Could you check a few things on this drawing? It's one solid part, dimensions in mm from its lowest x, y, z. Round coordinates to 2 decimals unless told otherwise and drop trailing zeros. Write each loop counter-clockwise with the first axis right and the second up, starting at its lowest first coordinate (ties: lowest second). Pieces come first, ordered by that corner, then holes. Notation, with made-up numbers: (26, 24.25) -> (43, 24.25) arc R25 ccw to (43, 44.25) -> close; hole circle Ø3 at (-37.5, -1). An arc over 180 degrees is marked (long way). Answer in a Markdown table with one row per item.
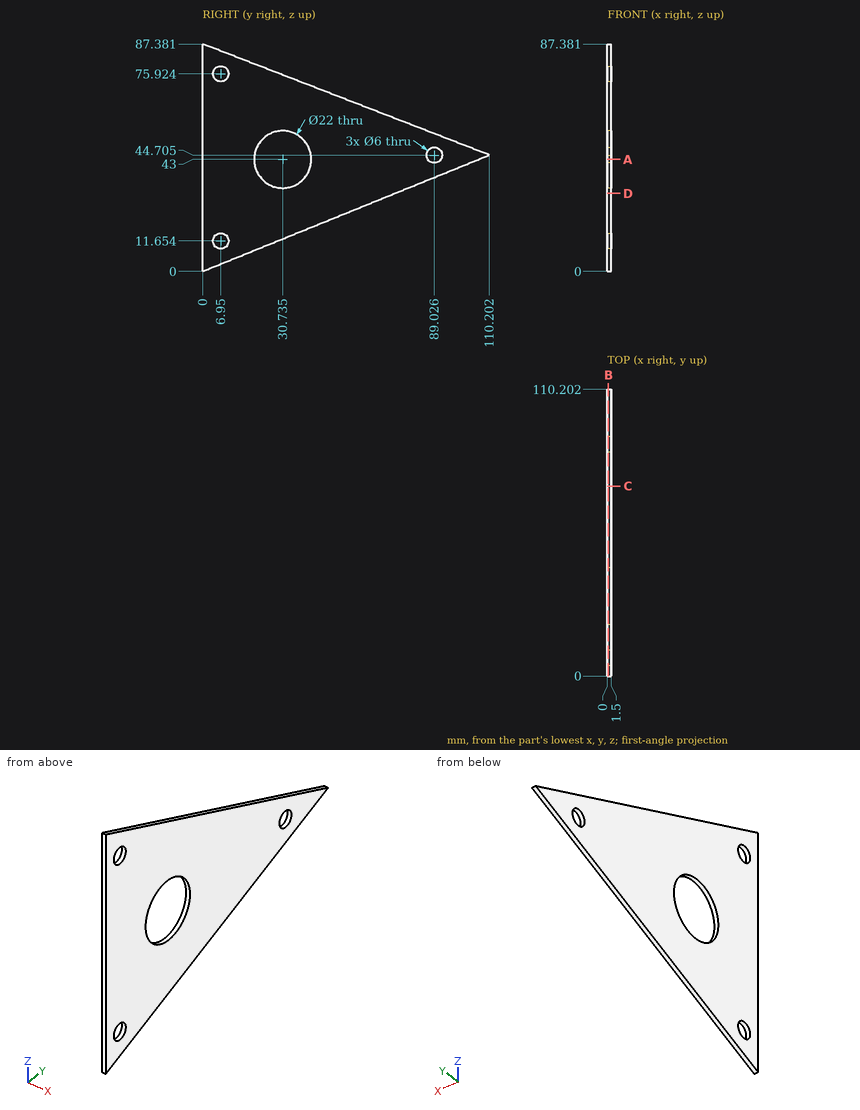
1) Imagine slicing it at D-D, the plane z = 30. Please give me the cut outline in (x, y).
Findings:
| item | result |
|---|---|
| outline | (0, 0) -> (1.5, 0) -> (1.5, 73.95) -> (0, 73.95) -> close |
2) Imagine slicing it at A-A, the plane z = 43. Please give me the cut outline in (x, y) (1 decimal).
Findings:
| item | result |
|---|---|
| outline | (0, 0) -> (1.5, 0) -> (1.5, 19.7) -> (0, 19.7) -> close; (0, 41.7) -> (1.5, 41.7) -> (1.5, 86.6) -> (0, 86.6) -> close; (0, 91.5) -> (1.5, 91.5) -> (1.5, 106) -> (0, 106) -> close |
3) Imagine slicing it at B-B, the plane x = 0.4. Count the separate pieces of the cut face and the enclosed holes in it, plus the area to 3 significant figures.
Findings:
| item | result |
|---|---|
| separate pieces | 1 |
| enclosed holes | 4 |
| area | 4,350 mm^2 |
4) Imagine slicing it at C-C, the plane y = 73. Please give me the cut outline in (x, z).
Findings:
| item | result |
|---|---|
| outline | (0, 29.61) -> (1.5, 29.61) -> (1.5, 59.11) -> (0, 59.11) -> close |
5) For pin 1 (8 mm diameter, centred on y = 6.95, z = 11.65, fed in from +X), with a flat end and sliding along its axis, tell me the tip position at first contact or that it passes through.
Findings:
| item | result |
|---|---|
| pin 1 | stops at x = 1.5 |
6) Please list where these lines run through material, in increasing order: line 1 (Z direction, x = 0.65, y = 6) (1 decimal); line 2 (Z direction, x = 0.7, y = 27.5) (1 decimal); line 3 (Z direction, x = 1.3, y = 89.5).
Findings:
| item | result |
|---|---|
| line 1 | z = 2.4 to 8.8, 14.5 to 73.1, 78.8 to 85.1 |
| line 2 | z = 11.2 to 32.5, 53.5 to 76.7 |
| line 3 | z = 36.31 to 41.74, 47.67 to 52.72 |
